```python
from build123d import *

# Parameters (mm, degrees)
SKETCH1_W           = 30
SKETCH1_H           = 30
BOSS_EXTRUDE1_DEPTH = 30
SKETCH2_R           = 5
CUT_EXTRUDE1_DEPTH  = 15


with BuildPart() as part:
    # Sketch1 → Boss-Extrude1 (new body)
    with BuildSketch(Plane(origin=(0, 0, 0), x_dir=(1, 0, 0), z_dir=(0, 1, 0))):
        with Locations((15, 15)):
            Rectangle(SKETCH1_W, SKETCH1_H)
    extrude(amount=BOSS_EXTRUDE1_DEPTH)

    # Sketch2 → Cut-Extrude1 (cut)
    with BuildSketch(Plane(origin=(30, 0, 0), x_dir=(0, 0, -1), z_dir=(1, 0, 0))):
        with Locations((15, 15)):
            Circle(SKETCH2_R)
    extrude(amount=-CUT_EXTRUDE1_DEPTH, mode=Mode.SUBTRACT)

    # Sketch4 → Cut-Revolve1 (revolve, cut)
    with BuildSketch(Plane(origin=(15, 0, 0), x_dir=(0, 0, -1), z_dir=(1, 0, 0))):
        with BuildLine():
            Line((25, 15), (5, 15))
            ThreePointArc((5, 15), (15, 5), (25, 15))
        make_face()
    revolve(axis=Axis((15, 15, -25), (0, 0, 1)), mode=Mode.SUBTRACT)


solid = part.part
```
Can you work these out from the model? Positions are in its coordinate system, mm. Coordinates: 2 decimals unless noted, no trailing zeros. Order: outer loops, then holes, each group sorted by start corner. A loop starts at its lowest first (then second) coordinate and runs counter-clockwise, first axis right, second up.
1. If we section it at A-A (y = 15): Please give me the cut outline in (x, z).
2. If we section it at D-D (z = -6.75): Please give me the cut outline in (x, y), then the cut area to 3 significant figures.
3. If we section it at C-C (y = 7): Please give me the cut outline in (x, z).
4. Thinking about a two-plate mould opening in Z: for faces 1 (the face through (15, 15, 0)), 2 (the face through (15, 15, -30)), 3 (the face through (15, 0, -15)), 4 (the face through (26.875, 10.564, -17.307)), which applies, +Z half, -Z half, draft (parallel to the pull), parting line (faces both ways), or undercut?
5. If we section it at B-B (z = -15): Please give me the cut outline in (x, y), then the cut area to 3 significant figures.
6. I need wall thicknesses on line 1 (Y direction, x = 26, z = -15); line 2 (Z direction, x = 28.5, y = 15); line 3 (Z direction, x = 10, y = 18.5). Which ranges of each line are inside material? Lowest first, please.
Entries:
1. outline: (0, -30) - (30, -30) - (30, -20) - (23.66, -20) arc R10 cw (long way) to (23.66, -10) - (30, -10) - (30, 0) - (0, 0) - close
2. outline: (0, 0) - (30, 0) - (30, 30) - (0, 30) - close; hole circle Ø11.3 at (15, 15)
2. area: 800 mm2
3. outline: (0, -30) - (30, -30) - (30, 0) - (0, 0) - close; hole circle Ø12 at (15, -15)
4. face 1: +Z half
4. face 2: -Z half
4. face 3: draft
4. face 4: undercut
5. outline: (0, 0) - (30, 0) - (30, 10) - (23.66, 10) arc R10 cw (long way) to (23.66, 20) - (30, 20) - (30, 30) - (0, 30) - close
5. area: 532 mm2
6. line 1: y = 0 to 10, 20 to 30
6. line 2: z = -30 to -20, -10 to 0
6. line 3: z = -30 to -22.92, -7.08 to 0
